from build123d import *

# Parameters (mm, degrees)
BOSS_EXTRU_1_DEPTH      = 504
ENL_V_MAT_EXTRU_1_DEPTH = 590
ENL_V_MAT_EXTRU_2_DEPTH = 590
ENL_V_MAT_EXTRU_3_DEPTH = 41
ENL_V_MAT_EXTRU_4_DEPTH = 41


with BuildPart() as part:
    # Esquisse1 → Boss.-Extru.1 (new body)
    with BuildSketch(Plane(origin=(0, 0, 0), x_dir=(1, 0, 0), z_dir=(0, 1, 0))):
        Polygon((-20, 20.113636364), (20, 20.113636364), (20, 18.113636364), (-18, 18.113636364), (-18, -19.886363636), (-20, -19.886363636), align=None)
    extrude(amount=BOSS_EXTRU_1_DEPTH)

    # Esquisse2 → Enlèv. mat.-Extru.1 (cut)
    with BuildSketch(Plane(origin=(0, 0, -20.113636364), x_dir=(-1, 0, 0), z_dir=(0, 0, -1))):
        Polygon((20, 0), (-20, 40), (-20, 0), align=None)
    extrude(amount=-ENL_V_MAT_EXTRU_1_DEPTH, mode=Mode.SUBTRACT)

    # Esquisse3 → Enlèv. mat.-Extru.2 (cut)
    with BuildSketch(Plane.ZY.offset(20)):
        Polygon((-20.113636364, 0), (19.886363636, 40), (19.886363636, 0), align=None)
    extrude(amount=-ENL_V_MAT_EXTRU_2_DEPTH, mode=Mode.SUBTRACT)

    # Esquisse4 → Enlèv. mat.-Extru.3 (cut, through all)
    with BuildSketch(Plane.ZY.offset(20)):
        Polygon((-20.113636364, 504), (19.886363636, 464), (19.886363636, 504), align=None)
    extrude(amount=-ENL_V_MAT_EXTRU_3_DEPTH, mode=Mode.SUBTRACT)

    # Esquisse5 → Enlèv. mat.-Extru.4 (cut, through all)
    with BuildSketch(Plane(origin=(0, 0, -20.113636364), x_dir=(-1, 0, 0), z_dir=(0, 0, -1))):
        Polygon((20, 504), (-20, 464), (-20, 504), align=None)
    extrude(amount=-ENL_V_MAT_EXTRU_4_DEPTH, mode=Mode.SUBTRACT)


solid = part.part
The listing builds one solid part. Answer for the finished solid, in the listing's coordinates (mm). A direction names the side the tool comes from. Round coordinates to 2 decimals unless told otherwise and drop trailing zeros. Write each loop counter-clockwise with the first axis right and the second up, starting at its lowest first coordinate (ties: lowest second). Pieces come first, ordered by that corner, then holes. Notation, with made-up numbers: (-22, -7) - (12, -7) arc R22 ccw to (12, 0) - close; hole circle Ø7 at (-24.5, 26.25). An arc over 180 degrees is marked (long way). Use a Markdown table: item, result. Add a question column.
1. Flat-ended cylindrical pins translate along their axes: P1, Ø11.5, axis at x = 9, y = 219, coming from the +Z side; P2, Ø8, axis at y = 91, z = 14.5, coming from the +X side. Find the tip coordinate at first contact, or state that the pin passes through.
2. The part is cut by section B-B (x = -7). Write down the section's boundary in (y, z), and give its area (3 significant figures).
3. The part is cut by section A-A (y = 113.5). Write down the section's boundary in (x, z).
4. Consider line 1 (Z direction, x = 16.5, y = 376); line 2 (X direction, y = 248.5, z = 16.5); line 3 (X direction, y = 474, z = -18.5). Determine where each line is inside the solid, lowest interval first.
5. A tool of negligible diameter and unlimited length cuts with its end or side. For faces 1 (the face through (1, 248, -18.114)), 2 (the face through (0, 248, -20.114)), from which of +Z, -Z, +X, -X, +Y, -Y can it reach the whole face along a straight path? Write none if from no direction.
6. The part is cut by section C-C (z = 13.5). Write down the section's boundary in (x, y), and give its area (3 significant figures).
Reported:
| question | item | result |
|---|---|---|
| 1 | P1 | z = -18.11 |
| 1 | P2 | x = -18 |
| 2 | outline | (13, -20.11) - (491, -20.11) - (491, -18.11) - (13, -18.11) - close |
| 2 | area | 956 mm^2 |
| 3 | outline | (-20, -20.11) - (20, -20.11) - (20, -18.11) - (-18, -18.11) - (-18, 19.89) - (-20, 19.89) - close |
| 4 | line 1 | -20.11 to -18.11 |
| 4 | line 2 | -20 to -18 |
| 4 | line 3 | -20 to 10 |
| 5 | face 1 | +Z, +X, +Y, -Y |
| 5 | face 2 | -Z, +X, -X, +Y, -Y |
| 6 | outline | (-20, 33.61) - (-18, 33.61) - (-18, 470.39) - (-20, 470.39) - close |
| 6 | area | 874 mm^2 |
